from build123d import *

# Parameters (mm, degrees)
SKETCH1_R           = 4
SKETCH1_R_2         = 2
BOSS_EXTRUDE1_DEPTH = 5
CUT_EXTRUDE1_DEPTH  = 5
SKETCH3_W           = 4
SKETCH3_H           = 1
CUT_EXTRUDE2_DEPTH  = 5


with BuildPart() as part:
    # Sketch1 → Boss-Extrude1 (new body)
    with BuildSketch(Plane.XY):
        Circle(SKETCH1_R)
        Circle(SKETCH1_R_2, mode=Mode.SUBTRACT)
    extrude(amount=BOSS_EXTRUDE1_DEPTH)

    # Sketch2 → Cut-Extrude1 (cut)
    with BuildSketch(Plane(origin=(0, 0, 0), x_dir=(1, 0, 0), z_dir=(0, 1, 0))):
        Polygon((-4, -2), (0, -2), (0, -3), (4, -3), (4, -5), (-4, -5), align=None)
    extrude(amount=CUT_EXTRUDE1_DEPTH, mode=Mode.SUBTRACT)

    # Sketch3 → Cut-Extrude2 (cut)
    with BuildSketch(Plane(origin=(0, 0, 0), x_dir=(1, 0, 0), z_dir=(0, 1, 0))):
        with Locations((-2, -4.5)):
            Rectangle(SKETCH3_W, SKETCH3_H)
    extrude(amount=-CUT_EXTRUDE2_DEPTH, mode=Mode.SUBTRACT)


solid = part.part
Can you work these out from the model? Positions are in its coordinate system, mm. A direction names the side the tool comes from. Coordinates: 2 decimals unless noted, no trailing zeros. Write each loop counter-clockwise with the first axis right and the second up, starting at its lowest first coordinate (ties: lowest second). Pieces come first, ordered by that corner, then holes. Notation, with made-up numbers: (19, 14) -> (69, 14) arc R20 cw to (69, 39) -> close; hole circle Ø1 at (22, 8.25). An arc over 180 degrees is marked (long way). Write each question's results on one line, items separated by ' | '. Start each with the question number.
Q1. Imagine slicing it at B-B (y = -0.5). Write out the boundary of the cut face in (x, z).
Q2. We'd pull the mould along Y, two halves only. Please class faces 4 (the face through (1.846, -3.549, 1.909)), 5 (the face through (0.923, -1.774, 1.909)), 6 (the face through (3, 0, 4)), 7 (the face through (2, 2, 3)): +Y half, -Y half, draft (parallel to the pull), parting line (faces both ways), or undercut.
Q3. Imagine slicing it at A-A (x = -1.5). Write out the boundary of the cut face in (y, z).
Q4. On a 3-axis mill with a long thin cutter (end or side, diameter ignored), from which of +Z, -Z, +X, -X, +Y, -Y can I reach the whole of each face in a straight line? I mean faces 1 (the face through (-2, -1, 0)), 2 (the face through (-2, -2, 4)), 3 (the face through (-3, 0, 3)). Say none if no direction works.
Q5. Imagine slicing it at C-C (z = 1.8). Write out the boundary of the cut face in (x, y).
Q6. Imagine slicing it at D-D (y = 2.75). Write out the boundary of the cut face in (x, z).
Q7. If I drill on probe 1 along X at (y, z) = (0, 1); probe 2 along Z at (x, y) = (-1.75, 3.5), over which ranges is the centre line in solid material (lowest first)?
Q8. I'm going to push flat-ended pins straight in: pin 1 (3 mm diameter, centred on x = -3, y = -2.5, fed in from +Z); pin 2 (4.5 mm diameter, centred on x = -1, y = 2.5, fed in from +Z); pin 3 (1 mm diameter, centred on x = 3, z = 4.5, fed in from +Y). Where does each tip first touch, or does it pass through?
Taken from the geometry:
1) outline: (-3.97, 0) -> (-1.94, 0) -> (-1.94, 4) -> (-3.97, 4) -> close; (1.94, 0) -> (3.97, 0) -> (3.97, 5) -> (1.94, 5) -> close
2) face 4: parting line | face 5: undercut | face 6: +Y half | face 7: draft
3) outline: (-3.71, 0) -> (-1.32, 0) -> (-1.32, 4) -> (-3.71, 4) -> close; (1.32, 0) -> (3.71, 0) -> (3.71, 2) -> (1.32, 2) -> close
4) face 1: -Z, +X, -X, +Y, -Y | face 2: +Z, -X, +Y, -Y | face 3: +Z, -X, +Y
5) outline: circle Ø8 at (0, 0); hole circle Ø4 at (0, 0)
6) outline: (-2.9, 0) -> (2.9, 0) -> (2.9, 3) -> (0, 3) -> (0, 2) -> (-2.9, 2) -> close
7) probe 1: x = -4 to -2, 2 to 4 | probe 2: z = 0 to 2
8) pin 1: stops at z = 4 | pin 2: stops at z = 3 | pin 3: stops at y = 0
